from build123d import *

# Parameters (mm, degrees)
BASE_EXTRUDE_DEPTH = 101.6
SLOT_DEPTH         = 127.877735455
LPATTERN1_COUNT    = 2
LPATTERN1_PITCH    = 50.8


with BuildPart() as part:
    # Sketch1 → Base-Extrude (new body)
    with BuildSketch(Plane.XY):
        with BuildLine():
            Line((17.6403, 16.339286512), (19.729882578, 19.063533504))
            ThreePointArc((19.729882578, 19.063533504), (19.156045845, 20.609744632), (17.6403, 21.2598))
            Line((17.6403, 21.2598), (14.70327367, 21.2598))
            ThreePointArc((14.70327367, 21.2598), (13.223883481, 20.647016519), (12.6111, 19.16762633))
            Line((12.6111, 19.16762633), (12.6111, 15.61465))
            Line((12.6111, 15.61465), (11.1125, 15.61465))
            Line((11.1125, 15.61465), (11.1125, 19.16762633))
            ThreePointArc((11.1125, 19.16762633), (12.164213258, 21.706686742), (14.70327367, 22.7584))
            Line((14.70327367, 22.7584), (17.6403, 22.7584))
            ThreePointArc((17.6403, 22.7584), (20.415434554, 21.446284653), (21.162428673, 18.4688666))
            Line((21.162428673, 18.4688666), (19.1389, 15.830735923))
            Line((19.1389, 15.830735923), (19.1389, 10.749129415))
            Line((19.1389, 10.749129415), (20.6375, 9.0662125))
            Line((20.6375, 9.0662125), (20.6375, -4.8244125))
            Line((20.6375, -4.8244125), (19.1389, -6.507329415))
            Line((19.1389, -6.507329415), (19.1389, -13.358784555))
            Line((19.1389, -13.358784555), (20.553458003, -14.773342558))
            ThreePointArc((20.553458003, -14.773342558), (18.729942105, -18.270236732), (15.019825564, -16.932883251))
            ThreePointArc((15.019825564, -16.932883251), (13.000752562, -16.523120627), (12.480559153, -18.5166))
            Line((12.480559153, -18.5166), (-12.480559153, -18.5166))
            ThreePointArc((-12.480559153, -18.5166), (-13.000752562, -16.523120627), (-15.019825564, -16.932883251))
            ThreePointArc((-15.019825564, -16.932883251), (-18.729942105, -18.270236732), (-20.553458003, -14.773342558))
            Line((-20.553458003, -14.773342558), (-19.1389, -13.358784555))
            Line((-19.1389, -13.358784555), (-19.1389, -6.507329415))
            Line((-19.1389, -6.507329415), (-20.6375, -4.8244125))
            Line((-20.6375, -4.8244125), (-20.6375, 9.0662125))
            Line((-20.6375, 9.0662125), (-19.1389, 10.749129415))
            Line((-19.1389, 10.749129415), (-19.1389, 15.830735923))
            Line((-19.1389, 15.830735923), (-21.162428673, 18.4688666))
            ThreePointArc((-21.162428673, 18.4688666), (-20.415434554, 21.446284653), (-17.6403, 22.7584))
            Line((-17.6403, 22.7584), (-14.70327367, 22.7584))
            ThreePointArc((-14.70327367, 22.7584), (-12.164213258, 21.706686742), (-11.1125, 19.16762633))
            Line((-11.1125, 19.16762633), (-11.1125, 15.61465))
            Line((-11.1125, 15.61465), (-12.6111, 15.61465))
            Line((-12.6111, 15.61465), (-12.6111, 19.16762633))
            ThreePointArc((-12.6111, 19.16762633), (-13.223883481, 20.647016519), (-14.70327367, 21.2598))
            Line((-14.70327367, 21.2598), (-17.6403, 21.2598))
            ThreePointArc((-17.6403, 21.2598), (-19.156045845, 20.609744632), (-19.729882578, 19.063533504))
            Line((-19.729882578, 19.063533504), (-17.6403, 16.339286512))
            Line((-17.6403, 16.339286512), (-17.6403, 10.17860201))
            Line((-17.6403, 10.17860201), (-19.1389, 8.495685095))
            Line((-19.1389, 8.495685095), (-19.1389, -4.253885095))
            Line((-19.1389, -4.253885095), (-17.6403, -5.93680201))
            Line((-17.6403, -5.93680201), (-17.6403, -13.979525))
            Line((-17.6403, -13.979525), (-19.1389, -15.478125))
            ThreePointArc((-19.1389, -15.478125), (-18.092238669, -16.906954381), (-16.414285827, -16.33992034))
            ThreePointArc((-16.414285827, -16.33992034), (-13.428073412, -14.819877156), (-10.898992189, -17.018))
            Line((-10.898992189, -17.018), (10.898992189, -17.018))
            ThreePointArc((10.898992189, -17.018), (13.323359075, -14.834630878), (16.30518861, -16.15877141))
            ThreePointArc((16.30518861, -16.15877141), (17.990302879, -16.935279743), (19.1389, -15.478125))
            Line((19.1389, -15.478125), (17.6403, -13.979525))
            Line((17.6403, -13.979525), (17.6403, -5.93680201))
            Line((17.6403, -5.93680201), (19.1389, -4.253885095))
            Line((19.1389, -4.253885095), (19.1389, 8.495685095))
            Line((19.1389, 8.495685095), (17.6403, 10.17860201))
            Line((17.6403, 10.17860201), (17.6403, 16.339286512))
        make_face()
    extrude(amount=BASE_EXTRUDE_DEPTH)

    # Sketch2 → Slot (cut, through all)
    with BuildSketch(Plane(origin=(-0.093451067, -18.5166, -16.466077999), x_dir=(1, 0, 0), z_dir=(0, -1, 0))):
        with BuildLine():
            Line((7.237201067, 53.772327999), (7.237201067, 39.484827999))
            ThreePointArc((7.237201067, 39.484827999), (0.093451067, 32.341077999), (-7.050298933, 39.484827999))
            Line((-7.050298933, 39.484827999), (-7.050298933, 53.772327999))
            ThreePointArc((-7.050298933, 53.772327999), (0.093451067, 60.916077999), (7.237201067, 53.772327999))
        make_face()
    slot = extrude(amount=-SLOT_DEPTH, mode=Mode.SUBTRACT)

    # LPattern1: Slot ×2
    with Locations(*[(0, 0, i * LPATTERN1_PITCH) for i in range(1, LPATTERN1_COUNT)]):
        add(slot, mode=Mode.SUBTRACT)


solid = part.part
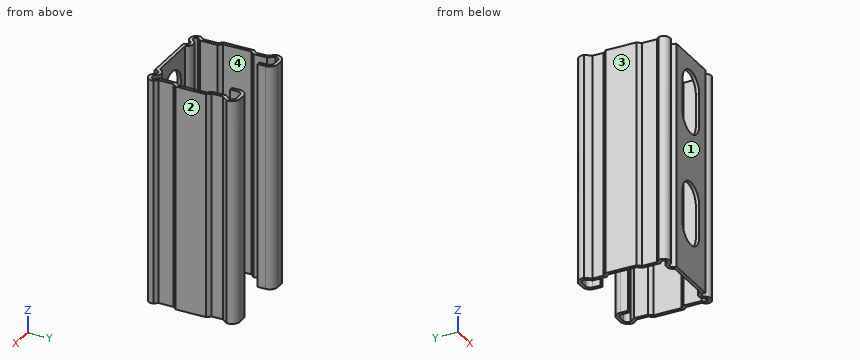
Build history of the part. All positions in model axes, mm. Face numbers are marked on the shaded views. Coordinates: 2 decimals unless noted, no trailing zeros. Order: outer loops, then holes, each group sorted by start corner. A loop starts at its lowest first (then second) coordinate and runs counter-clockwise, first axis right, second up. Notation, with made-up numbers: (71.25, 38) - (116.25, 38) arc R15 ccw to (116.25, 66) - close; hole circle Ø2 at (-28.5, 19.25). An arc over 180 degrees is marked (long way). Write item = value, one per line. Start each with the question number.
1) Saw through at C-C on x = 9.5. Write the cut outline in (y, z).
2) Saw through at A-A on x = 0. Write the cut outline in (y, z) (3 decimals).
3) Two-plate mould, pull along X, no slides. Class the marked faces 1, 2, 3 and 4: pulls with the +X half, pulls with the -X half, needs draft (parallel to the pull), parting line crosses it, or undercut.
4) Flat gauge pins, fed straight in: pin 1 Ø11 at (y, z) = (5, 34.5) entering from +X; pin 2 Ø1.8 at (y, z) = (16.5, 33.5) entering from +X; pin 3 Ø1.6 at (y, z) = (-18, 29.5) entering from -X; pin 4 Ø12 at (x, y) = (10, 16) entering from +Z. Where does each tip first touch, or does it go through?
5) Wall check: line 1 along X through (y, z) = (5.5, 26.5); line 2 along X through (y, z) = (14.5, 50); line 3 along X through (y, z) = (18, 58). Give the ranges that are in metal, low to high. Write a range as from..to.
6) Saw through at B-B on y = 3. Write the cut outline in (x, z), then the cut area to 3 significant figures.
From the geometry:
q1.outline = (-18.52, 0) - (-17.02, 0) - (-17.02, 101.6) - (-18.52, 101.6) - close
q2.outline = (-18.517, 0) - (-17.018, 0) - (-17.018, 15.875) - (-18.517, 15.875) - close; (-18.517, 44.45) - (-17.018, 44.45) - (-17.018, 66.675) - (-18.517, 66.675) - close; (-18.517, 95.25) - (-17.018, 95.25) - (-17.018, 101.6) - (-18.517, 101.6) - close
q3.face_1 = needs draft
q3.face_2 = pulls with the +X half
q3.face_3 = pulls with the -X half
q3.face_4 = undercut
q4.pin_1 = 20.64
q4.pin_2 = 20.34
q4.pin_3 = -20.09
q4.pin_4 = 101.6
q5.line_1 = -20.64..-19.14, 19.14..20.64
q5.line_2 = -19.14..-17.64, 17.64..19.14
q5.line_3 = -20.8..-18.91, -12.61..-11.11, 11.11..12.61, 18.91..20.8
q6.outline = (-20.64, 0) - (-19.14, 0) - (-19.14, 101.6) - (-20.64, 101.6) - close; (19.14, 0) - (20.64, 0) - (20.64, 101.6) - (19.14, 101.6) - close
q6.area = 305 mm^2
